Can you work these out from the model? Positions are in its coordinate system, mm. Give positions to 0.01 mm unless a question says otherwise; leave off trailing zeros. Write each loop counter-clockwise with the first axis right and the second up, starting at its lowest first coordinate (ties: lowest second). Pieces come first, ordered by that corner, then holes. Notation, with made-up numbers: (72.5, -13) -> (113.5, -13) arc R9 cw to (113.5, -2) -> close; hole circle Ø10 at (75, 37). An arc over 180 degrees is marked (long way). Answer as CSV lines item,"result". Start each with the question number.
1. If we section it at C-C on z = 0.5: Write out the boundary of the cut face in (x, y).
2. I need wall thicknesses on line 1 (Y direction, x = 2, z = 0.2); line 2 (X direction, y = -36, z = 0.1); line 3 (X direction, y = -24.5, z = 0.2). Which ranges of each line are inside material? Lowest first, please. Write a range as [from, to].
3. If we section it at B-B on y = -8: Write out the boundary of the cut face in (x, z).
4. I'm going to push flat-ended pins straight in: P1, Ø8, axis at x = 0, y = 30.5, coming from the +Z side; P2, Ø3, axis at x = 30.5, y = 0, coming from the +Z side. Where does each tip first touch, or does it pass through?
5. If we section it at A-A on x = 0: Write out the boundary of the cut face in (y, z), plus the area to 3 significant figures.
6. If we section it at D-D on x = -24.5: Write out the boundary of the cut face in (y, z) (3 decimals).
```python
from build123d import *

# Parameters (mm, degrees)
SKETCH1_R           = 2.5
BOSS_EXTRUDE1_DEPTH = 0.8


with BuildPart() as part:
    # Sketch1 → Boss-Extrude1 (new body)
    with BuildSketch(Plane.XY):
        with BuildLine():
            Line((-35, 0), (-35, -35))
            ThreePointArc((-35, -35), (0, -70), (35, -35))
            Line((35, -35), (35, 0))
            ThreePointArc((35, 0), (0, 35), (-35, 0))
        make_face()
        with Locations((-30.5, 0)):
            Circle(SKETCH1_R, mode=Mode.SUBTRACT)
        with Locations((0, 30.5)):
            Circle(SKETCH1_R, mode=Mode.SUBTRACT)
        with Locations((30.5, 0)):
            Circle(SKETCH1_R, mode=Mode.SUBTRACT)
        with Locations((0, -65.5)):
            Circle(SKETCH1_R, mode=Mode.SUBTRACT)
        with Locations((-30.5, -35)):
            Circle(SKETCH1_R, mode=Mode.SUBTRACT)
        with Locations((30.5, -35)):
            Circle(SKETCH1_R, mode=Mode.SUBTRACT)
        with BuildLine():
            Line((-26, 0), (-26, -35))
            ThreePointArc((-26, -35), (0, -61), (26, -35))
            Line((26, -35), (26, 0))
            ThreePointArc((26, 0), (0, 26), (-26, 0))
        make_face(mode=Mode.SUBTRACT)
    extrude(amount=BOSS_EXTRUDE1_DEPTH)


solid = part.part
```
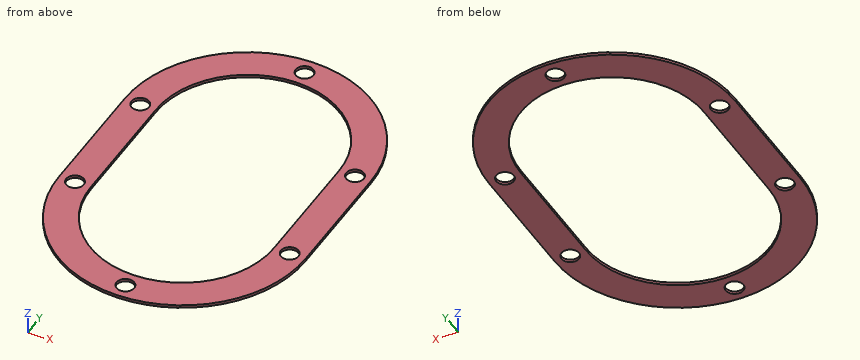
Computed values:
1,outline,"(-35, -35) arc R35 ccw to (35, -35) -> (35, 0) arc R35 ccw to (-35, 0) -> close; hole circle Ø5 at (-30.5, -35); hole circle Ø5 at (-30.5, 0); hole (-26, -35) arc R26 ccw to (26, -35) -> (26, 0) arc R26 ccw to (-26, 0) -> close; hole circle Ø5 at (0, -65.5); hole circle Ø5 at (0, 30.5); hole circle Ø5 at (30.5, -35); hole circle Ø5 at (30.5, 0)"
2,line 1,"y = [-69.94, -67], [-64, -60.92], [25.92, 29], [32, 34.94]"
2,line 2,"x = [-34.99, -32.79], [-28.21, -25.98], [25.98, 28.21], [32.79, 34.99]"
2,line 3,"x = [-35, -26], [26, 35]"
3,outline,"(-35, 0) -> (-26, 0) -> (-26, 0.8) -> (-35, 0.8) -> close; (26, 0) -> (35, 0) -> (35, 0.8) -> (26, 0.8) -> close"
4,P1,"stops at z = 0.8"
4,P2,"passes through"
5,outline,"(-70, 0) -> (-68, 0) -> (-68, 0.8) -> (-70, 0.8) -> close; (-63, 0) -> (-61, 0) -> (-61, 0.8) -> (-63, 0.8) -> close; (26, 0) -> (28, 0) -> (28, 0.8) -> (26, 0.8) -> close; (33, 0) -> (35, 0) -> (35, 0.8) -> (33, 0.8) -> close"
5,area,"6.40 mm2"
6,outline,"(-59.995, 0) -> (-43.703, 0) -> (-43.703, 0.8) -> (-59.995, 0.8) -> close; (8.703, 0) -> (24.995, 0) -> (24.995, 0.8) -> (8.703, 0.8) -> close"
